```python
from build123d import *

# Parameters (mm, degrees)
CUT_EXTRUDE_1_DEPTH = 48.053161424
EXTRUDE_1_DEPTH     = 8


with BuildPart() as part:
    # Sketch 1 → Revolve 1 (revolve)
    with BuildSketch(Plane(origin=(0, 0, 0), x_dir=(0, 0, -1), z_dir=(1, 0, 0)), mode=Mode.PRIVATE) as revolve_1_sk:
        with BuildLine():
            Line((0, 23), (-16, 23))
            Line((-16, 23), (-18, 21))
            Line((-18, 21), (-18, 18))
            Line((-18, 18), (-16, 16))
            Line((-16, 16), (-16, 0))
            Line((-16, 0), (-14.334262465, 0))
            Line((-14.334262465, 0), (-6, 0))
            Line((-6, 0), (-6, 4))
            add(Edge.make_bspline(
                [(-12, 10), (-11.486384316, 10), (-7.521156143, 9.156929615), (-6, 5.021272174), (-6, 4)],
                knots=[0, 0, 0, 0, 0.351628705, 1, 1, 1, 1], degree=3))
            Line((-12, 10), (-12, 13.5))
            Line((-12, 13.5), (-8, 17.5))
            Line((-8, 17.5), (18, 17.5))
            Line((18, 17.5), (18, 21))
            Line((18, 21), (16, 23))
            Line((16, 23), (0, 23))
        make_face()
    revolve(revolve_1_sk.sketch.rotate(Axis((0, 0, 28.673920663), (0, 0, -1)), 90), axis=Axis((0, 0, 28.673920663), (0, 0, -1)))

    # Sketch 2 → Cut-Extrude 1 (cut, through all)
    with BuildSketch(Plane.XY.offset(16)):
        with BuildLine():
            Line((1.125, -0.953939201), (1.125, 0.953939201))
            ThreePointArc((1.125, 0.953939201), (-1.475, 0), (1.125, -0.953939201))
        make_face()
    extrude(amount=-CUT_EXTRUDE_1_DEPTH, mode=Mode.SUBTRACT)

    # Sketch 3 → Cut-Revolve 1 (revolve, cut)
    with BuildSketch(Plane(origin=(0, 0, 0), x_dir=(0, 0, -1), z_dir=(1, 0, 0)), mode=Mode.PRIVATE) as cut_revolve_1_sk:
        Polygon((18, 21), (16, 23), (14, 23), (14, 21), (11, 21), (11, 23), (-11, 23), (-11, 21), (-14, 21), (-14, 23), (-16, 23), (-18, 21), (-18, 24.334722486), (18, 24.334722486), align=None)
    revolve(cut_revolve_1_sk.sketch.rotate(Axis((0, 0, 27.637589676), (0, 0, -1)), 90), axis=Axis((0, 0, 27.637589676), (0, 0, -1)), mode=Mode.SUBTRACT)

    # Sketch 4 → Extrude 1 (add, symmetric)
    with BuildSketch(Plane.XY):
        with BuildLine():
            Line((-3.5, 22.732135843), (-5.592854337, 24.132135843))
            Line((-5.592854337, 24.132135843), (3.5, 22.732135843))
            ThreePointArc((3.5, 22.732135843), (0, 23), (-3.5, 22.732135843))
        make_face()
        with BuildLine():
            Line((2.99811261, 24.589658818), (11.063772532, 20.164149805))
            ThreePointArc((11.063772532, 20.164149805), (7.866463296, 21.612930278), (4.485924186, 22.558290808))
            Line((4.485924186, 22.558290808), (2.99811261, 24.589658818))
        make_face()
        with BuildLine():
            Line((11.227462929, 22.081306034), (17.293090813, 15.164069709))
            ThreePointArc((17.293090813, 15.164069709), (14.784115023, 17.619022192), (11.930779711, 19.663582977))
            Line((11.930779711, 19.663582977), (11.227462929, 22.081306034))
        make_face()
        with BuildLine():
            Line((18.102615519, 16.909621857), (21.436607123, 8.334979008))
            ThreePointArc((21.436607123, 8.334979008), (19.918584287, 11.5), (17.936607123, 14.397156835))
            Line((17.936607123, 14.397156835), (18.102615519, 16.909621857))
        make_face()
        with BuildLine():
            Line((22.794325512, 9.698387725), (22.994552243, 0.500566828))
            ThreePointArc((22.994552243, 0.500566828), (22.650578319, 3.993908086), (21.779014999, 7.394221099))
            Line((21.779014999, 7.394221099), (22.794325512, 9.698387725))
        make_face()
        with BuildLine():
            Line((24.736703439, 1.3173849), (21.779014999, -7.394221099))
            ThreePointArc((21.779014999, -7.394221099), (22.650578319, -3.993908086), (22.994552243, -0.500566828))
            Line((22.994552243, -0.500566828), (24.736703439, 1.3173849))
        make_face()
        with BuildLine():
            Line((23.695469857, -7.222513986), (17.936607123, -14.397156835))
            ThreePointArc((17.936607123, -14.397156835), (19.918584287, -11.5), (21.436607123, -8.334979008))
            Line((21.436607123, -8.334979008), (23.695469857, -7.222513986))
        make_face()
        with BuildLine():
            Line((19.796212902, -14.891271093), (11.930779711, -19.663582977))
            ThreePointArc((11.930779711, -19.663582977), (14.784115023, -17.619022192), (17.293090813, -15.164069709))
            Line((17.293090813, -15.164069709), (19.796212902, -14.891271093))
        make_face()
        with BuildLine():
            Line((13.50924051, -20.763921134), (4.485924186, -22.558290808))
            ThreePointArc((4.485924186, -22.558290808), (7.866463296, -21.612930278), (11.063772532, -20.164149805))
            Line((11.063772532, -20.164149805), (13.50924051, -20.763921134))
        make_face()
        with BuildLine():
            Line((5.592854337, -24.132135843), (-3.5, -22.732135843))
            ThreePointArc((-3.5, -22.732135843), (0, -23), (3.5, -22.732135843))
            Line((3.5, -22.732135843), (5.592854337, -24.132135843))
        make_face()
        with BuildLine():
            Line((-2.99811261, -24.589658818), (-11.063772532, -20.164149805))
            ThreePointArc((-11.063772532, -20.164149805), (-7.866463296, -21.612930278), (-4.485924186, -22.558290808))
            Line((-4.485924186, -22.558290808), (-2.99811261, -24.589658818))
        make_face()
        with BuildLine():
            Line((-11.227462929, -22.081306034), (-17.293090813, -15.164069709))
            ThreePointArc((-17.293090813, -15.164069709), (-14.784115023, -17.619022192), (-11.930779711, -19.663582977))
            Line((-11.930779711, -19.663582977), (-11.227462929, -22.081306034))
        make_face()
        with BuildLine():
            Line((-18.102615519, -16.909621857), (-21.436607123, -8.334979008))
            ThreePointArc((-21.436607123, -8.334979008), (-19.918584287, -11.5), (-17.936607123, -14.397156835))
            Line((-17.936607123, -14.397156835), (-18.102615519, -16.909621857))
        make_face()
        with BuildLine():
            Line((-22.794325512, -9.698387725), (-22.994552243, -0.500566828))
            ThreePointArc((-22.994552243, -0.500566828), (-22.650578319, -3.993908086), (-21.779014999, -7.394221099))
            Line((-21.779014999, -7.394221099), (-22.794325512, -9.698387725))
        make_face()
        with BuildLine():
            Line((-24.736703439, -1.3173849), (-21.779014999, 7.394221099))
            ThreePointArc((-21.779014999, 7.394221099), (-22.650578319, 3.993908086), (-22.994552243, 0.500566828))
            Line((-22.994552243, 0.500566828), (-24.736703439, -1.3173849))
        make_face()
        with BuildLine():
            Line((-23.695469857, 7.222513986), (-17.936607123, 14.397156835))
            ThreePointArc((-17.936607123, 14.397156835), (-19.918584287, 11.5), (-21.436607123, 8.334979008))
            Line((-21.436607123, 8.334979008), (-23.695469857, 7.222513986))
        make_face()
        with BuildLine():
            Line((-19.796212902, 14.891271093), (-11.930779711, 19.663582977))
            ThreePointArc((-11.930779711, 19.663582977), (-14.784115023, 17.619022192), (-17.293090813, 15.164069709))
            Line((-17.293090813, 15.164069709), (-19.796212902, 14.891271093))
        make_face()
        with BuildLine():
            Line((-13.50924051, 20.763921134), (-4.485924186, 22.558290808))
            ThreePointArc((-4.485924186, 22.558290808), (-7.866463296, 21.612930278), (-11.063772532, 20.164149805))
            Line((-11.063772532, 20.164149805), (-13.50924051, 20.763921134))
        make_face()
    extrude(amount=EXTRUDE_1_DEPTH, both=True)


solid = part.part
```
The model under review builds one solid part; all positions refer to its coordinate system, in mm. A direction names the side the tool comes from. Round coordinates to 2 decimals unless told otherwise and drop trailing zeros. Write each loop counter-clockwise with the first axis right and the second up, starting at its lowest first coordinate (ties: lowest second). Pieces come first, ordered by that corner, then holes. Notation, with made-up numbers: M 22,-6.5 L 26,-6.5 A20 cw 26,10.5 Z; hole C 87.5,41.5 d4. An arc over 180 degrees is marked long. Use CSV: the item, a comma, the result in double quotes. Start each with the question number.
(1) We need section A-A, the plane z = -13. State the section outline as (x, y) points.
(2) Tool access review of faces 4 (the face through (-20.856, 10.76, -0.112)), 5 (the face through (-13.1, -19.4, 8)), 6 (the face through (-2, 0, 6)): name each direction out of +Z, -Z, +X, -X, +Y, -Y from which nothing blocks a thin tool from reaching the whole face with its end or side.
(3) For line 1 along Y through (x, z) = (2.5, 7); line 2 along Y through (x, z) = (0, 10) (3 decimals); line 3 along Y through (x, z) = (0, 13.75) (3 decimals), list the stretches that pass through material, from the lowest coordinate up.
(4) Clearance check with flat-ended pins moving along their axes: P1, Ø1.9, axis at x = -7.5, y = 21.5, coming from the -Z side; P2, Ø2, axis at y = -15, z = 13.5, coming from the -X side; P3, Ø6.5, axis at x = -14.5, y = -17.5, coming from the +Z side; P4, Ø5, axis at y = 14, z = 12.5, coming from the -X side. State where each tip first meets the part, or that it passes through.
(5) The part is to be moulded in two halves that separate along Y. For faces 1 (the face through (2.4, -23.3, 8)), 2 (the face through (9, 5, 12)), 3 (the face through (-2.994, -22.804, 15.014)), say which applies: +Y half, -Y half, draft (parallel to the pull), parting line (faces both ways), or undercut.
Findings:
1,outline,"C 0,0 d42; hole C 0,0 d35"
2,face 4,"+Z, -Z, -X"
2,face 5,"+Z, -X, -Y"
2,face 6,"-Z"
3,line 1,"-23.66 to -17.32, -6.38 to 6.38, 17.32 to 22.89"
3,line 2,"-23 to -15.5, -9.513 to -1.475, 1.475 to 9.513, 15.5 to 23"
3,line 3,"-21 to -1.475, 1.475 to 21"
4,P1,"z = -17.18"
4,P2,"x = -18.14"
4,P3,"z = 18"
4,P4,"x = -19.62"
5,face 1,"draft"
5,face 2,"undercut"
5,face 3,"parting line"
